```python
from build123d import *

# Parameters (mm, degrees)
F0_W     = 104
F0_H     = 50.8
F1_DEPTH = 6.35
F2_W     = 104
F2_H     = 44.45
F3_DEPTH = 6.35
F6_D     = 18.25625
F8_DEPTH = 50.801
F9_DEPTH = 50.801


# Not quite as in the source:
# - a length typed as a fraction of an inch, garbled in the dataset ("3 / 203.2 mm" for 3/8 in), is restored


with BuildPart() as f1:
    # F0 (on Front) → F1 (new body)
    with BuildSketch(Plane.XZ):
        Rectangle(F0_W, F0_H)
    extrude(amount=F1_DEPTH)

    # F2 (on face) → F3 (join)
    with BuildSketch(Plane.XY.offset(25.4)):
        with Locations((0, -28.575)):
            Rectangle(F2_W, F2_H)
    extrude(amount=-F3_DEPTH)

    # F6 (through all)
    with Locations(Plane.XY.offset(25.4)):
        with Locations((0, -28.575)):
            Hole(F6_D / 2)

    # F7 (on face) → F8 (cut, through all)
    with BuildSketch(Plane.XY.offset(25.4)):
        with BuildLine():
            Line((-29.775, -19.05), (-52, -19.05))
            Line((-52, -19.05), (-52, -50.8))
            Line((-52, -50.8), (-20.25, -50.8))
            Line((-20.25, -50.8), (-20.25, -28.575))
            ThreePointArc((-20.25, -28.575), (-23.0398079092, -21.8398079092), (-29.775, -19.05))
        make_face()
        with BuildLine():
            Line((20.25, -28.575), (20.25, -50.8))
            Line((20.25, -50.8), (52, -50.8))
            Line((52, -50.8), (52, -19.05))
            Line((52, -19.05), (29.775, -19.05))
            ThreePointArc((29.775, -19.05), (23.0398079092, -21.8398079092), (20.25, -28.575))
        make_face()
    extrude(amount=-F8_DEPTH, mode=Mode.SUBTRACT)

    # F4 (on face) → F9 (cut, through all)
    with BuildSketch(Plane(origin=(0, 0, 0), x_dir=(-1, 0, 0), z_dir=(0, 1, 0))):
        with BuildLine():
            ThreePointArc((37.9072132349, -18.4), (40.2884632349, -20.78125), (42.6697132349, -18.4))
            Line((42.6697132349, -18.4), (42.6697132349, 7.05))
            ThreePointArc((42.6697132349, 7.05), (40.2884632349, 9.43125), (37.9072132349, 7.05))
            Line((37.9072132349, 7.05), (37.9072132349, -18.4))
        make_face()
        with BuildLine():
            ThreePointArc((-42.6697132349, -18.4), (-40.2884632349, -20.78125), (-37.9072132349, -18.4))
            Line((-37.9072132349, -18.4), (-37.9072132349, 7.05))
            ThreePointArc((-37.9072132349, 7.05), (-40.2884632349, 9.43125), (-42.6697132349, 7.05))
            Line((-42.6697132349, 7.05), (-42.6697132349, -18.4))
        make_face()
    extrude(amount=-F9_DEPTH, mode=Mode.SUBTRACT)


solid = f1.part
```
The model under review builds one solid part; all positions refer to its coordinate system, in mm. A direction names the side the tool comes from. Give positions to 0.01 mm unless a question says otherwise; leave off trailing zeros. Write each loop counter-clockwise with the first axis right and the second up, starting at its lowest first coordinate (ties: lowest second). Pieces come first, ordered by that corner, then holes. Notation, with made-up numbers: M 33.25,74 L 60.25,74 A28 ccw 60.25,100 Z; hole C -32,35.5 d7. An arc over 180 degrees is marked long. Answer in a Markdown table with one row per item.
Item 1: Add section C-C on y = -30.5. Give the boundary of the cut face in (x, z), plus the area to 3 significant figures.
Check sheet entries:
| item | result |
|---|---|
| outline | M -20.25,19.05 L -8.92,19.05 L -8.92,25.4 L -20.25,25.4 Z; M 8.92,19.05 L 20.25,19.05 L 20.25,25.4 L 8.92,25.4 Z |
| area | 144 mm2 |
Item 2: Add section D-D on z = 22. Give the boundary of the cut face in (x, y) (3 decimals).
Check sheet entries:
| item | result |
|---|---|
| outline | M -52,-19.05 L -29.775,-19.05 A9.525 cw -20.25,-28.575 L -20.25,-50.8 L 20.25,-50.8 L 20.25,-28.575 A9.525 cw 29.775,-19.05 L 52,-19.05 L 52,0 L -52,0 Z; hole C 0,-28.575 d18.256 |
Item 3: Draft analysis for pull direction X (two halves, no side actions). For faces 1 (the face through (-20.25, -40, 22)), 2 (the face through (-1, 0, 0)), 3 (the face through (-42.67, -3, -6)), 4 (the face through (37.907, -3, -6)), state which applies: +X half, -X half, draft (parallel to the pull), parting line (faces both ways), or undercut.
Check sheet entries:
| item | result |
|---|---|
| face 1 | -X half |
| face 2 | draft |
| face 3 | undercut |
| face 4 | undercut |
Item 4: For P1, Ø22, axis at x = -15, y = -18, coming from the -Z side; P2, Ø3, axis at y = -45, z = 22, coming from the -X side; P3, Ø5, axis at x = -44.5, z = 21, coming from the -Y side, all flat-tipped, find the tip position at first contact; note any pin that passes through.
Check sheet entries:
| item | result |
|---|---|
| P1 | z = 19.05 |
| P2 | x = -20.25 |
| P3 | y = -19.05 |
Item 5: Tool access review of faces 5 (the face through (-4.91, -20.88, 22.18)), 6 (the face through (-40.34, -3.13, 9.43)), 7 (the face through (-41, -19.05, 22)), 8 (the face through (41, -19.05, 22)), 9 (the face through (0, -50.8, 22)): name each direction out of +Z, -Z, +X, -X, +Y, -Y from which nothing blocks a thin tool from reaching the whole face with its end or side.
Check sheet entries:
| item | result |
|---|---|
| face 5 | +Z, -Z |
| face 6 | +Y, -Y |
| face 7 | +Z, -Z, -X, -Y |
| face 8 | +Z, -Z, +X, -Y |
| face 9 | +Z, -Z, +X, -X, -Y |
Item 6: Add section A-A on x = 0. Give the boundary of the cut face in (y, z).
Check sheet entries:
| item | result |
|---|---|
| outline | M -50.8,19.05 L -37.7,19.05 L -37.7,25.4 L -50.8,25.4 Z; M -19.45,19.05 L -6.35,19.05 L -6.35,-25.4 L 0,-25.4 L 0,25.4 L -19.45,25.4 Z |
Item 7: For line 1 along X through (y, z) = (-4.5, -12.5); line 2 along Y through (x, z) = (0, 22.25); line 3 along Y through (x, z) = (-7, -2), list the stretches that pass through material, from the lowest coordinate up.
Check sheet entries:
| item | result |
|---|---|
| line 1 | -52 to -42.67, -37.91 to 37.91, 42.67 to 52 |
| line 2 | -50.8 to -37.7, -19.45 to 0 |
| line 3 | -6.35 to 0 |
Item 8: Add section B-B on z = -6.5. Give the boundary of the cut face in (x, y), plus the area to 3 significant figures.
Check sheet entries:
| item | result |
|---|---|
| outline | M -52,-6.35 L -42.67,-6.35 L -42.67,0 L -52,0 Z; M -37.91,-6.35 L 37.91,-6.35 L 37.91,0 L -37.91,0 Z; M 42.67,-6.35 L 52,-6.35 L 52,0 L 42.67,0 Z |
| area | 600 mm2 |
